Autodesk Inventor part; units mm, degrees
ref_plane "YZ Plane" through (0, 0, 0) normal (1, 0, 0) x (0, 1, 0)
ref_plane "XZ Plane" through (0, 0, 0) normal (0, 1, 0) x (-1, 0, 0)
ref_plane "XY Plane" through (0, 0, 0) normal (0, 0, 1) x (1, 0, 0)
sketch "Sketch1" plane through (0, 0, 0) normal (0, 0, 1) x (1, 0, 0)
  line L0 (45.8511, 50) -> (65.8511, 50)
  line L1 (65.8511, 50) -> (65.8511, -50)
  line L2 (65.8511, -50) -> (45.8511, -50)
  line L3 (45.8511, -50) -> (45.8511, 50)
  line L4 (45.8511, 50) -> (65.8511, -50) construction
  line L5 (65.8511, 50) -> (45.8511, -50) construction
  line L6 (100.8511, 74.3) -> (100.8511, -74.3)
  point P0 (0, 0)
  point P1 (55.8511, 0)
  point P2 (55.8511, 0)
  dimension "d0" = 100
  dimension "d1" = 20
  dimension "d36" = 45
extrude "Plate1" add sketch "Sketch1" along normal blind 1.2
sketch "Sketch2" plane through (65.8511, -48.9608, 0.6) normal (0, -0.8660254, -0.5) x (1, 0, 0)
  line L0 (-20, 0) -> (0, 0)
  line L1 (0, 0) -> (0, 12)
  line L2 (0, 12) -> (-20, 12)
  line L3 (-20, 12) -> (-20, 0)
edge flange "Flange1" height 12 angle 60 thickness 1.2 bend radius 1.2 thickness toward (0, -0.8660254, -0.5) relief tear relief width 1.2 relief depth 0.6 corner gap 1.2 corner form 0 edges at (55.8511, -50, 1.2) (55.8511, 50, 1.2) wall of the first edge with corners at (45.8511, -48.9608, 0.6) (65.8511, -48.9608, 0.6) (65.8511, -54.9608, 10.9923) (45.8511, -54.9608, 10.9923)
bend "Bend1"
corner "Corner1"
sketch "Sketch3" plane through (45.8511, -54.9608, 9.7923) normal (0, 0, 1) x (1, 0, 0)
  line L0 (20, 0) -> (0, 0)
  line L1 (0, 0) -> (0, -18)
  line L2 (0, -18) -> (20, -18)
  line L3 (20, -18) -> (20, 0)
edge flange "Flange2" height 18 angle 60 thickness 1.2 bend radius 1.2 thickness toward (0, 0, 1) relief tear relief width 1.2 relief depth 0.6 corner gap 1.2 corner form 0 edges at (55.8511, -56, 10.3923) (55.8511, 56, 10.3923) wall of the first edge with corners at (65.8511, -54.9608, 9.7923) (45.8511, -54.9608, 9.7923) (45.8511, -72.9608, 9.7923) (65.8511, -72.9608, 9.7923)
bend "Bend2"
corner "Corner2"
chamfer "Corner Chamfer1" distance 4 angle 45 4 edges at (45.8511, -72.9608, 10.3923) (65.8511, -72.9608, 10.3923) (45.8511, 72.9608, 10.3923) (65.8511, 72.9608, 10.3923)
sketch "Sketch4" plane through (45.8511, -56.3464, 10.9923) normal (0, 0, 1) x (1, 0, 0)
  line L0 (4, 129.3072) -> (16, 129.3072)
  line L1 (16, -16.6144) -> (4, -16.6144)
  point P0 (-45.8511, 56.3464)
  point P1 (10, -10.6144)
  point P2 (10, 123.3072)
  point P3 (10, 129.3072)
  point P4 (10, -16.6144)
  dimension "d27" = 6
  dimension "d28" = 6
hole "Hole1" at (55.8511, -66.9608, 10.9923) at (55.8511, 66.9608, 10.9923) direction (0, 0, -1) diameter 4.2 depth 1.2 tip angle 118
equation "\"d34\" = Thickness"
equation "\"d4\" = BendReliefWidth"
equation "\"d5\" = BendReliefDepth"
equation "\"d6\" = MinimumRemnant"
equation "\"d7\" = BendRadius"
equation "\"d10\" = BendRadius"
equation "\"d11\" = CornerReliefSize"
equation "\"d12\" = GapSize"
equation "\"d13\" = JacobiRadiusSize"
equation "\"d14\" = BendReliefWidth"
equation "\"d15\" = BendReliefDepth"
equation "\"d16\" = MinimumRemnant"
equation "\"d17\" = BendRadius"
equation "\"d20\" = BendRadius"
equation "\"d21\" = CornerReliefSize"
equation "\"d22\" = GapSize"
equation "\"d23\" = JacobiRadiusSize"
equation "\"BendRadius\" = Thickness"
equation "\"BendReliefWidth\" = Thickness"
equation "\"BendReliefDepth\" = 0.5 * Thickness"
equation "\"CornerReliefSize\" = 4 * Thickness"
equation "\"MinimumRemnant\" = 2 * Thickness"
equation "\"TransitionRadius\" = BendRadius"
equation "\"JacobiRadiusSize\" = BendRadius"
equation "\"GapSize\" = Thickness"
equation "\"d3\" = BendRadius"
Here's how the part is built. I have some questions about the finished solid (model axes, mm). A direction names the side the tool comes from. Give positions to 0.01 mm unless a question says otherwise; leave off trailing zeros. Loops run counter-clockwise (first coordinate to the right, second up) from the corner with the lowest first, then second, coordinate; pieces in that order, holes last. Notation, with made-up numbers: (-13.5, -17.5) -> (-2.5, -17.5) arc R24 ccw to (-2.5, 8.5) -> close; hole circle Ø3 at (53.25, 5). An arc over 180 degrees is marked (long way). Answer as a JSON object with one key per item and string values. Group by question number.
Item 1: On a 3-axis mill with a long thin cutter (end or side, diameter ignored), from which of +Z, -Z, +X, -X, +Y, -Y can I reach the whole of each face in a straight line? I mean faces 1 (the flat face through (56, 1, 1.2)), 2 (the flat face through (55.7, -64.5, 9.792)), 3 (the flat face through (56, 64.5, 9.792)), 4 (the flat face through (47.88, -70.99, 10.4)). Say none if no direction works.
Item 2: Thinking about a two-plate mould opening in X: for faces 5 (the cylindrical face through (53.77, 67.23, 10.38)), 6 (the flat face through (56, 63, 10.992)), 7 (the flat face through (47.88, 70.99, 10.38)), 8 (the cylindrical face through (54.432, -65.413, 10.384)), which applies, pulls with the +X half, pulls with the -X half, needs draft (parallel to the pull), parting line crosses it, or undercut?
Item 3: Imagine slicing it at B-B on y = -8. Write out the boundary of the cut face in (x, z), then the cut area to 3 significant figures.
Item 4: I need wall thicknesses on L1, parallel to Z at x = 52.5, y = 25; L2, parallel to Z at x = 53.5, y = 57.5; L3, parallel to Y at x = 56, z = 3.5. Which ranges of each line are inside material? Lowest first, please.
Item 5: Imagine slicing it at A-A on z = 7.25. Write out the boundary of the cut face in (x, y).
Item 6: Imagine slicing it at C-C on y = 53. Write out the boundary of the cut face in (x, z).
Item 7: Will these pins go through, and if not, where does the flat tip stop? pin 1 (6 mm diameter, centred on x = 58, y = 16, fed in from +Z); pin 2 (5 mm diameter, centred on x = 50.5, z = 3, fed in from -Y); pin 3 (5 mm diameter, centred on x = 55.85, y = 66.96, fed in from -Z).
Answer list:
{
 "1": {"face 1": "+Z, +X, -X", "face 2": "-Z, +X, -X, -Y", "face 3": "-Z, +X, -X, +Y", "face 4": "+Z, -Z, -X, -Y"},
 "2": {"face 5": "undercut", "face 6": "needs draft", "face 7": "pulls with the -X half", "face 8": "undercut"},
 "3": {"outline": "(45.85, 0) -> (65.85, 0) -> (65.85, 1.2) -> (45.85, 1.2) -> close", "area": "24.0 mm2"},
 "4": {"L1": "z = 0 to 1.2", "L2": "z = 9.79 to 10.99", "L3": "y = -52.02 to -50.64, 50.64 to 52.02"},
 "5": {"outline": "(45.85, -54.19) -> (65.85, -54.19) -> (65.85, -52.8) -> (45.85, -52.8) -> close; (45.85, 52.8) -> (65.85, 52.8) -> (65.85, 54.19) -> (45.85, 54.19) -> close"},
 "6": {"outline": "(45.85, 5.2) -> (65.85, 5.2) -> (65.85, 7.6) -> (45.85, 7.6) -> close"},
 "7": {"pin 1": "stops at z = 1.2", "pin 2": "stops at y = -53.18", "pin 3": "stops at z = 9.79"}
}
